```python
from build123d import *

# Parameters (mm, degrees)
BOSS_EXTRU_1_DEPTH           = 5
ENL_V_MAT_EXTRU_1_DEPTH      = 131.1355063
ENL_V_MAT_EXTRU_1_DEPTH_BACK = 140
ESQUISSE2_R                  = 3.5
D_GAGEMENT_M51_D             = 5.8
D_GAGEMENT_M51_DEPTH         = 90
D_GAGEMENT_M51_TIP           = 1.742495795
ENL_V_MAT_EXTRU_3_DEPTH      = 167.883192683
ENL_V_MAT_EXTRU_3_DEPTH_BACK = 167.883192683
ESQUISSE6_R                  = 6.5
ENL_V_START                  = -0.5
ESQUISSE7_W                  = 75
ESQUISSE7_H                  = 4
ENL_V_MAT_EXTRU_4_DEPTH      = 0.5


with BuildPart() as part:
    # Esquisse1 → Boss.-Extru.1 (new body)
    with BuildSketch(Plane.XY):
        with BuildLine():
            Line((-20, 56.568542495), (-73.333333333, 37.712361663))
            ThreePointArc((-73.333333333, 37.712361663), (-100, 0), (-73.333333333, -37.712361663))
            Line((-73.333333333, -37.712361663), (-20, -56.568542495))
            ThreePointArc((-20, -56.568542495), (34.641016151, -48.989794856), (60, 0))
            ThreePointArc((60, 0), (34.641016151, 48.989794856), (-20, 56.568542495))
        make_face()
    extrude(amount=BOSS_EXTRU_1_DEPTH)

    # Esquisse2 → Enlèv. mat.-Extru.1 (cut, two sides: drawn at the far end of the back side and taken through both)
    with BuildSketch(Plane(origin=(15, 0, -5.5), x_dir=(0, -1, 0), z_dir=(0, 0, -1)).offset(-ENL_V_MAT_EXTRU_1_DEPTH_BACK)):
        with Locations(Location((-22.5, 15, 0), (0, 0, 90))):
            Circle(ESQUISSE2_R)
        with Locations(Location((22.5, 15, 0), (0, 0, 90))):
            Circle(ESQUISSE2_R)
        with Locations(Location((22.5, 75, 0), (0, 0, 90))):
            Circle(ESQUISSE2_R)
        with Locations(Location((-22.5, 75, 0), (0, 0, 90))):
            Circle(ESQUISSE2_R)
    extrude(amount=ENL_V_MAT_EXTRU_1_DEPTH + ENL_V_MAT_EXTRU_1_DEPTH_BACK, mode=Mode.SUBTRACT)

    # Dégagement M51
    with Locations(Plane(origin=(15, 0, 48), x_dir=(0, 1, 0), z_dir=(0, 0, 1))):
        with Locations((43.604918173, 41.666666667), (0, -35), (-43.301270189, -10), (43.301270189, -10), (-22.360679775, 95), (22.360679775, 95), (-43.604918173, 41.666666667)):
            Hole(D_GAGEMENT_M51_D / 2, depth=D_GAGEMENT_M51_DEPTH)
            with Locations((0, 0, -(D_GAGEMENT_M51_DEPTH + D_GAGEMENT_M51_TIP / 2))):  # 118° drill point
                Cone(0, D_GAGEMENT_M51_D / 2, D_GAGEMENT_M51_TIP, mode=Mode.SUBTRACT)

    # Esquisse6 → Enlèv. mat.-Extru.3 (cut, two sides: drawn at the far end of the back side and taken through both)
    with BuildSketch(Plane(origin=(15, 0, -100), x_dir=(0, -1, 0), z_dir=(0, 0, -1)).offset(-ENL_V_MAT_EXTRU_3_DEPTH_BACK)):
        with Locations(Location((0, 15, 0), (0, 0, 180))):
            Circle(ESQUISSE6_R)
        with Locations(Location((0, 75, 0), (0, 0, 180))):
            Circle(ESQUISSE6_R)
    extrude(amount=ENL_V_MAT_EXTRU_3_DEPTH + ENL_V_MAT_EXTRU_3_DEPTH_BACK, mode=Mode.SUBTRACT)

    # Esquisse7 → Enlèv. mat.-Extru.4 (cut)
    with BuildSketch(Plane(origin=(15, 0, 0), x_dir=(0, -1, 0), z_dir=(0, 0, -1)).offset(ENL_V_START)):
        with Locations((0, -22.686269666)):
            Rectangle(ESQUISSE7_W, ESQUISSE7_H)
    extrude(amount=ENL_V_MAT_EXTRU_4_DEPTH, mode=Mode.SUBTRACT)


solid = part.part
```
Geometry check sheet. Reference: the model listing, model coordinates, mm. A direction names the side the tool comes from. Give positions to 0.01 mm unless a question says otherwise; leave off trailing zeros. Loops run counter-clockwise (first coordinate to the right, second up) from the corner with the lowest first, then second, coordinate; pieces in that order, holes last. Notation, with made-up numbers: M -20.75,39 L 22.25,39 A18 ccw 22.25,60 Z; hole C 38.5,46.25 d7. An arc over 180 degrees is marked long. Answer as CSV lines item,"result".
Item 1: Release check for a two-part mould opening along Y. For faces 1 (the flat face through (-21, 1, 5)), 2 (the cylindrical face through (-99.994, 0.689, 2.465)), 3 (the cylindrical face through (0, -19, 3)) record: pulls with the +Y half, pulls with the -Y half, needs draft (parallel to the pull), parting line crosses it, or undercut.
Values:
face 1,"needs draft"
face 2,"parting line crosses it"
face 3,"undercut"
Item 2: Cross-section at B-B on y = -22.5. Record the cut outline in (x, z).
Values:
outline,"M -93.07,0 L -82.9,0 L -82.9,5 L -93.07,5 Z; M -77.1,0 L -63.5,0 L -63.5,5 L -77.1,5 Z; M -56.5,0 L -3.5,0 L -3.5,5 L -56.5,5 Z; M 3.5,0 L 35.69,0 L 35.69,0.5 L 39.69,0.5 L 39.69,0 L 55.62,0 L 55.62,5 L 3.5,5 Z"
Item 3: Cross-section at A-A on x = 0. Record the cut outline in (y, z), and give its area (3 significant figures).
Values:
outline,"M -60,0 L -26,0 L -26,5 L -60,5 Z; M -19,0 L -6.5,0 L -6.5,5 L -19,5 Z; M 6.5,0 L 19,0 L 19,5 L 6.5,5 Z; M 26,0 L 60,0 L 60,5 L 26,5 Z"
area,"465 mm²"
Item 4: Material ranges on line 1 (X direction, y = 25, z = 0.8); line 2 (X direction, y = -22.5, z = 1.8); line 3 (Y direction, x = -5, z = 2.8), recorded low to high.
Values:
line 1,"x = -91.22 to -81.2, -78.8 to -62.45, -57.55 to -2.45, 2.45 to 54.54"
line 2,"x = -93.07 to -82.9, -77.1 to -63.5, -56.5 to -3.5, 3.5 to 55.62"
line 3,"y = -59.79 to -4.15, 4.15 to 59.79"
Item 5: Cross-section at D-D on z = 2.2. Count the separate pieces of the cut face and the enclosed holes in it, and give its area (3 significant figures).
Values:
separate pieces,"1"
enclosed holes,"13"
area,"13,900 mm²"
Item 6: Cross-section at C-C on x = 25. Record the cut outline in (y, z).
Values:
outline,"M -54.54,0 L -46.2,0 L -46.2,5 L -54.54,5 Z; M -40.4,0 L 40.4,0 L 40.4,5 L -40.4,5 Z; M 46.2,0 L 54.54,0 L 54.54,5 L 46.2,5 Z"
Item 7: Access from +Z, -Z, +X, -X, +Y, -Y to the whole of each face (thin tool, end or side, straight path). Record for faces 4 (the cylindrical face through (-56.503, -22.346, 2.535)), 5 (the flat face through (38, 1, 0.5)).
Values:
face 4,"+Z, -Z"
face 5,"-Z"
Item 8: Depth check by flat-ended pin: P1, Ø0.6, axis at x = 36.5, z = 0.5, coming from the +Y side; P2, Ø8, axis at x = -60, y = 0, coming from the -Z side; P3, Ø0.6, axis at y = -3, z = 0, coming from the -X side; P4, Ø1.2, axis at x = 37.5, y = -6, coming from the -Z side. Enter the tip coordinate at first touch or a pass-through.
Values:
P1,"stops at y = 47.85"
P2,"passes through"
P3,"stops at x = -99.91"
P4,"stops at z = 0.5"
